Source: CAD feature listing. Evaluate the final solid. Frame: model axes, mm. Face numbers are marked on the shaded views. Give positions to 0.01 mm unless a question says otherwise; leave off trailing zeros. Loops run counter-clockwise (first coordinate to the right, second up) from the corner with the lowest first, then second, coordinate; pieces in that order, holes last.
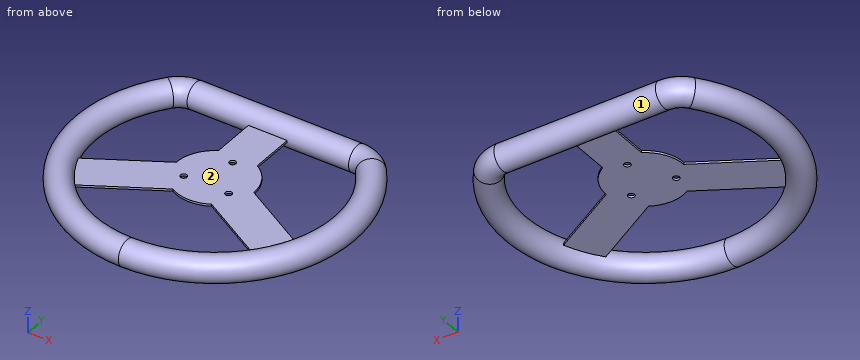
from build123d import *

# Parameters (mm, degrees)
F1_DEPTH = 0.8
F2_R     = 2.5
F3_DEPTH = 1.601
F5_R     = 10


with BuildPart() as f1:
    # F0 (on Top) → F1 (new body, symmetric)
    with BuildSketch(Plane.XY):
        with BuildLine():
            ThreePointArc((15, -25.9807621135), (25.9807621135, -15), (30, 0))
            ThreePointArc((30, 0), (25.9807621135, 15), (15, 25.9807621135))
            ThreePointArc((15, 25.9807621135), (0, 30), (-15, 25.9807621135))
            ThreePointArc((-15, 25.9807621135), (-25.9807621135, 15), (-30, 0))
            ThreePointArc((-30, 0), (-25.9807621135, -15), (-15, -25.9807621135))
            ThreePointArc((-15, -25.9807621135), (0, -30), (15, -25.9807621135))
        make_face()
        with BuildLine():
            Line((93.1227189477, -36.4439187764), (30, 0))
            ThreePointArc((30, 0), (25.9807621135, -15), (15, -25.9807621135))
            Line((15, -25.9807621135), (78.1227189477, -62.42468089))
            Line((78.1227189477, -62.42468089), (93.1227189477, -36.4439187764))
        make_face()
        with BuildLine():
            ThreePointArc((-15, 25.9807621135), (0, 30), (15, 25.9807621135))
            Line((15, 25.9807621135), (15, 70))
            Line((15, 70), (-15, 70))
            Line((-15, 70), (-15, 25.9807621135))
        make_face()
        with BuildLine():
            Line((-78.1227189477, -62.42468089), (-15, -25.9807621135))
            ThreePointArc((-15, -25.9807621135), (-25.9807621135, -15), (-30, 0))
            Line((-30, 0), (-93.1227189477, -36.4439187764))
            Line((-93.1227189477, -36.4439187764), (-78.1227189477, -62.42468089))
        make_face()
    extrude(amount=F1_DEPTH, both=True)

    # F2 (on face) → F3 (cut, through all)
    with BuildSketch(Plane.XY.offset(0.8)):
        with Locations((0, 20)):
            Circle(F2_R)
        with Locations((-17.3205080757, -10)):
            Circle(F2_R)
        with Locations((17.3205080757, -10)):
            Circle(F2_R)
    extrude(amount=-F3_DEPTH, mode=Mode.SUBTRACT)



with BuildPart() as f6:
    # F6: sweep along a path in F4
    with BuildLine(Plane.XY) as f6_path:
        Line((0, 70), (62.449979984, 70))
        ThreePointArc((62.449979984, 70), (71.1102340218, 68.0277563773), (78.06247498, 62.5))
        ThreePointArc((78.06247498, 62.5), (90.1387818866, -43.3012701892), (0, -100))
    # F5 (on Right) → F6 (sweep)
    with BuildSketch(Plane.YZ):
        with Locations((70, 0)):
            Circle(F5_R)
    sweep(path=f6_path.line)


with BuildPart() as f1_1:
    add(f1.part)

    add(f6.part)  # F7 merges F6
    # F7: F6 across plane
    add(f6.part.mirror(Plane.YZ))


solid = f1_1.part
1) Cut plane B-B (y = 20). State how many separate pieces and enclosed holes the cut face has, and give its area (3 significant figures).
Checks:
separate pieces: 4
enclosed holes: 0
area: 705 mm2
2) Ray query, probe 1 along Y at (x, z) = (0, 0.2); probe 2 along X at (y, z) = (53, -0.25); probe 3 along X at (y, z) = (-23, -2.25). Return the intervals inside material, ascending.
Checks:
probe 1: y = -110 to -90, -30 to 17.5, 22.5 to 80
probe 2: x = -96.39 to -72.74, -15 to 15, 72.74 to 96.39
probe 3: x = -107.31 to -87.28, 87.28 to 107.31
3) Contact query for flat-ended pins moving along their axis: P1, Ø1.5, axis at x = -73.5, z = -2.5, coming from the +Y side; P2, Ø1.3, axis at y = 35.5, z = -0.5, coming from the -X side; P3, Ø6.5, axis at x = -17.32, y = -10, coming from the +Z side. Output: stop coordinate, or through.
Checks:
P1: stops at y = 77.9
P2: stops at x = -104.32
P3: stops at z = 0.8
4) Pull-direction query (Y, two-part tool) for the marked faces 1 and 2; classes: released by +Y, released by -Y, zero draft, split by the parting line, or undercut.
Checks:
face 1: undercut
face 2: undercut
5) Cut plane A-A (z = -7.25). Return loops of the section in (x, y), and give its area (3 significant figures).
Checks:
outline: (-83.44, 66.8) arc R106.89 ccw (long way) to (83.44, 66.8) arc R26.89 ccw to (62.45, 76.89) - (-62.45, 76.89) arc R26.89 ccw to start; hole (-72.69, 58.2) arc R93.11 ccw (long way) to (72.69, 58.2) arc R13.11 ccw to (62.45, 63.11) - (-62.45, 63.11) arc R13.11 ccw to start
area: 8,400 mm2
